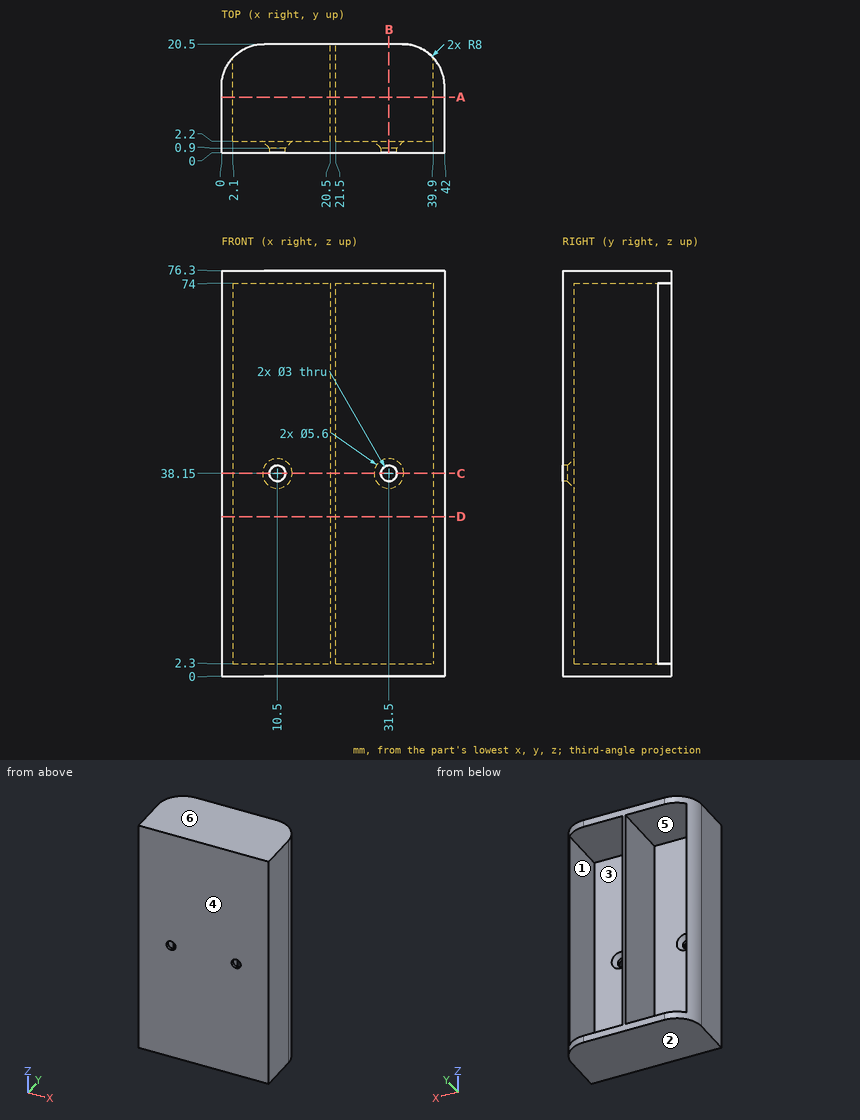
Answer from the drawing. Dimensions are ordinates in mm from the lowest x, y and z of the part. A direction names the side the tool comes from. Give positions to 0.01 mm unless a question says otherwise; leave off trailing zeros. Loops run counter-clockwise (first coordinate to the right, second up) from the corner with the lowest first, then second, coordinate; pieces in that order, holes last.
Item 1: For the marked faces 5 and 6, determine the directions among +Z, -Z, +X, -X, +Y, -Y from which every point of the face is accessible in a straight line to the end or side of a thin tool.
Item 2: The part is cut by section C-C (z = 38.15). Write down the section's boundary in (x, y), and give its area (3 significant figures).
Item 3: The part is cut by section A-A (y = 10.5). Write down the section's boundary in (x, z).
Item 4: The part is cut by section D-D (z = 30). Write down the section's boundary in (x, y), and give its area (3 significant figures).
Item 5: Each of these flat-tipped pins is pushed along its axis until it touches: pin 1 Ø12 at (x, z) = (10, 8.5) entering from +Y; pin 2 Ø20 at (x, z) = (8.5, 37.5) entering from +Y; pin 3 Ø5.5 at (y, z) = (15.5, 38.5) entering from -X; pin 4 Ø1.8 at (x, z) = (31.5, 38.15) entering from -Y. Where does it stop, or does it pass through?
Item 6: Find the intervals of material crossed by line 1 along X through (y, z) = (3.25, 65); line 2 along X through (y, z) = (0.45, 38.15); line 3 along Z through (x, y) = (13.5, 18.5), in increasing order.
Item 7: The mould has two halves that part along Z. Classify the marked faces 1, 2, 3 and 4: released by +Z, released by -Z, zero draft, split by the parting line, or undercut.
Item 8: The part is cut by section B-B (x = 31.5). Write down the section's boundary in (y, z), and give its area (3 significant figures).
Taken from the geometry:
1. face 5: +Y
1. face 6: +Z, +X, -X, +Y, -Y
2. outline: (0, 0) - (9, 0) - (9, 0.9) - (7.7, 2.2) - (2.1, 2.2) - (2.1, 17.9) arc R8 ccw to (0, 12.5) - close; (12, 0) - (30, 0) - (30, 0.9) - (28.7, 2.2) - (21.5, 2.2) - (21.5, 20.5) - (20.5, 20.5) - (20.5, 2.2) - (13.3, 2.2) - (12, 0.9) - close; (33, 0) - (42, 0) - (42, 12.5) arc R8 ccw to (39.9, 17.9) - (39.9, 2.2) - (34.3, 2.2) - (33, 0.9) - close
2. area: 153 mm2
3. outline: (0, 0) - (42, 0) - (42, 76.3) - (0, 76.3) - close; hole (2.1, 2.3) - (20.5, 2.3) - (20.5, 74) - (2.1, 74) - close; hole (21.5, 2.3) - (39.9, 2.3) - (39.9, 74) - (21.5, 74) - close
4. outline: (0, 0) - (42, 0) - (42, 12.5) arc R8 ccw to (39.9, 17.9) - (39.9, 2.2) - (21.5, 2.2) - (21.5, 20.5) - (20.5, 20.5) - (20.5, 2.2) - (2.1, 2.2) - (2.1, 17.9) arc R8 ccw to (0, 12.5) - close
4. area: 170 mm2
5. pin 1: stops at y = 2.2
5. pin 2: stops at y = 17.9
5. pin 3: stops at x = 0
5. pin 4: passes through
6. line 1: x = 0 to 2.1, 20.5 to 21.5, 39.9 to 42
6. line 2: x = 0 to 9, 12 to 30, 33 to 42
6. line 3: z = 0 to 2.3, 74 to 76.3
7. face 1: undercut
7. face 2: released by -Z
7. face 3: undercut
7. face 4: zero draft
8. outline: (0, 0) - (20.5, 0) - (20.5, 2.3) - (2.2, 2.3) - (2.2, 35.35) - (0.9, 36.65) - (0, 36.65) - close; (0, 39.65) - (0.9, 39.65) - (2.2, 40.95) - (2.2, 74) - (20.5, 74) - (20.5, 76.3) - (0, 76.3) - close
8. area: 244 mm2
